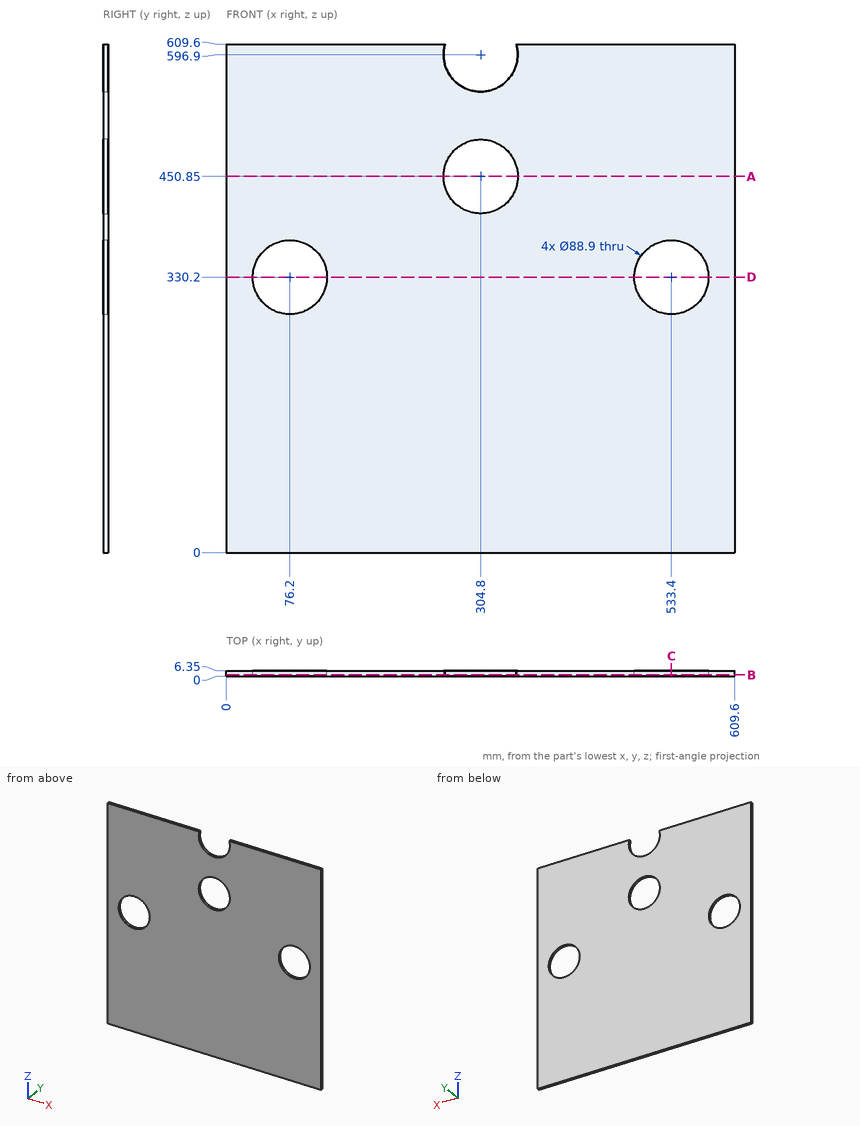
Here's the drawing with two shaded views (mm, measured from the low corner). I have some questions. Round coordinates to 2 decimals unless told otherwise and drop trailing zeros. Loops run counter-clockwise (first coordinate to the right, second up) from the corner with the lowest first, then second, coordinate; pieces in that order, holes last. Notation, with made-up numbers: M 86.25,24.5 L 109.25,24.5 A20 cw 109.25,58.5 Z; hole C 67.25,30 d4. An arc over 180 degrees is marked long. Put each result on its own line as item: value.
Q1. I need wall thicknesses on probe 1 along X at (y, z) = (5, 330.2); probe 2 along X at (y, z) = (4.5, 596.9); probe 3 along Z at (x, y) = (314, 5). Which ranges of each line are inside material? Lowest first, please.
Check result:
probe 1: 0 to 31.75, 120.65 to 488.95, 577.85 to 609.6
probe 2: 0 to 260.35, 349.25 to 609.6
probe 3: 0 to 407.36, 494.34 to 553.41
Q2. Imagine slicing it at C-C (x = 533.4). Write out the boundary of the cut face in (y, z).
Check result:
outline: M 0,0 L 6.35,0 L 6.35,285.75 L 0,285.75 Z; M 0,374.65 L 6.35,374.65 L 6.35,609.6 L 0,609.6 Z
Q3. Imagine slicing it at A-A (z = 450.85). Write out the boundary of the cut face in (x, y).
Check result:
outline: M 0,0 L 260.35,0 L 260.35,6.35 L 0,6.35 Z; M 349.25,0 L 609.6,0 L 609.6,6.35 L 349.25,6.35 Z
Q4. Imagine slicing it at D-D (z = 330.2). Write out the boundary of the cut face in (x, y).
Check result:
outline: M 0,0 L 31.75,0 L 31.75,6.35 L 0,6.35 Z; M 120.65,0 L 488.95,0 L 488.95,6.35 L 120.65,6.35 Z; M 577.85,0 L 609.6,0 L 609.6,6.35 L 577.85,6.35 Z
Q5. Imagine slicing it at B-B (y = 1.25). Write out the boundary of the cut face in (x, z), then the cut area to 3 significant figures.
Check result:
outline: M 0,0 L 609.6,0 L 609.6,609.6 L 347.4,609.6 A44.45 cw long 262.2,609.6 L 0,609.6 Z; hole C 76.2,330.2 d88.9; hole C 304.8,450.85 d88.9; hole C 533.4,330.2 d88.9
area: 349,000 mm2
